```python
from build123d import *

# Parameters (mm, degrees)
SKETCH1_R           = 10
BOSS_EXTRUDE1_DEPTH = 85
SCALE_1_SCALE       = 0.3
SKETCH_1_R          = 6
EXTRUDE_1_DEPTH     = 3
SKETCH_2_R          = 3
SKETCH_2_R_2        = 2.75
CUT_EXTRUDE_1_DEPTH = 25.5


with BuildPart() as part:
    # Sketch1 → Boss-Extrude1 (new body)
    with BuildSketch(Plane(origin=(0, 0, 0), x_dir=(1, 0, 0), z_dir=(0, 1, 0))):
        Circle(SKETCH1_R)
    extrude(amount=BOSS_EXTRUDE1_DEPTH)


with BuildPart() as part_1:
    # 축척1: scaled about (0, 42.5, 0)
    add(part.part.scale(SCALE_1_SCALE).moved(Location((0, 29.75, 0))))

    # 스케치1 → 보스-돌출1 (add)
    with BuildSketch(Plane(origin=(0, 55.25, 0), x_dir=(1, 0, 0), z_dir=(0, 1, 0))):
        Circle(SKETCH_1_R)
    extrude(amount=EXTRUDE_1_DEPTH)

    # 스케치2 → 컷-돌출1 (cut)
    with BuildSketch(Plane.XZ.offset(-29.75)):
        Circle(SKETCH_2_R)
        Circle(SKETCH_2_R_2, mode=Mode.SUBTRACT)
    extrude(amount=-CUT_EXTRUDE_1_DEPTH, mode=Mode.SUBTRACT)


solid = part_1.part
```
Source: CAD feature listing. Evaluate the final solid. Frame: model axes, mm. A direction names the side the tool comes from. Round coordinates to 2 decimals unless told otherwise and drop trailing zeros. Loops run counter-clockwise (first coordinate to the right, second up) from the corner with the lowest first, then second, coordinate; pieces in that order, holes last.
(1) Access query for faces 1 (the flat face through (0, 58.25, 0)), 2 (the flat face through (3, 55.25, 1)). Directions: +Z, -Z, +X, -X, +Y, -Y. A direction counts if a zero-diameter tool reaches every point of the face in a straight line with its end or side. Return the directions, or none.
From the geometry:
face 1: +Z, -Z, +X, -X, +Y
face 2: -Y
(2) Section query A-A (z = 0). Output: boundary loops of the cut face in (x, y), and give its area (3 significant figures).
From the geometry:
outline: (-6, 55.25) - (-2.75, 55.25) - (-2.75, 29.75) - (2.75, 29.75) - (2.75, 55.25) - (6, 55.25) - (6, 58.25) - (-6, 58.25) - close
area: 176 mm2
(3) Section query B-B (x = 0). Output: boundary loops of the cut face in (y, z).
From the geometry:
outline: (29.75, -2.75) - (55.25, -2.75) - (55.25, -6) - (58.25, -6) - (58.25, 6) - (55.25, 6) - (55.25, 2.75) - (29.75, 2.75) - close
(4) Contact query for flat-ended pins moving along their axis: pin 1 Ø4 at (x, z) = (-3, -3.5) entering from -Y; pin 2 Ø4 at (y, z) = (44.5, 0.5) entering from +X; pin 3 Ø6 at (y, z) = (44, -2) entering from -X. Output: stop coordinate, or through.
From the geometry:
pin 1: stops at y = 29.75
pin 2: stops at x = 2.75
pin 3: stops at x = -2.75
(5) Material intervals for probe 1 along Y at (x, z) = (3.75, 1); probe 2 along Z at (x, y) = (0.25, 56.75); probe 3 along X at (y, z) = (43.75, 0.25), sorted ascending.
From the geometry:
probe 1: y = 55.25 to 58.25
probe 2: z = -5.99 to 5.99
probe 3: x = -2.74 to 2.74
(6) Section query D-D (z = -3.5). Output: boundary loops of the cut face in (x, y).
From the geometry:
outline: (-4.87, 55.25) - (4.87, 55.25) - (4.87, 58.25) - (-4.87, 58.25) - close
(7) Section query C-C (y = 44). Output: boundary loops of the cut face in (x, z).
From the geometry:
outline: circle Ø5.5 at (0, 0)
